Part print with two shaded views. Sizes in mm from the minimum x, y, z corner. A direction names the side the tool comes from. Round coordinates to 2 decimals unless told otherwise and drop trailing zeros. Loops run counter-clockwise (first coordinate to the right, second up) from the corner with the lowest first, then second, coordinate; pieces in that order, holes last. Notation, with made-up numbers: M 23,79 L 33,79 A27 cw 33,112 Z; hole C -23.75,30 d5. An arc over 180 degrees is marked long. Use a Markdown table: item, result. Add a question column.
Item 1: Saw through at D-D on x = 1.5. Write the cut outline in (y, z).
Item 2: Saw through at C-C on x = 0.5. Write the cut outline in (y, z).
Item 3: Tool access for the marked faces 1, 2 and 3: list every direction of +Z, -Z, +X, -X, +Y, -Y with a clear straight run to the whole face (end or side of a thin tool).
Item 4: Saw through at A-A on y = 4. Write the cut outline in (x, z).
Item 5: Pin check, flat tips, straight feed: P1, Ø1.5, axis at x = 3, z = 7, coming from the +Y side; P2, Ø1.5, axis at x = 3.5, z = 2, coming from the +Y side; P3, Ø3.5, axis at y = 4, z = 3.5, coming from the -X side. Stop position of each tip, or through.
Item 6: Wall check: L1, parallel to Z at x = 7.65, y = 4; L2, parallel to Z at x = 1.75, y = 4; L3, parallel to Y at x = 6.5, z = 6 (1 decimal). Give the ranges that are in metal, low to high. Write a range as from..to.
Item 7: Two-plate mould, pull along Y, no slides. Class the marked faces 4, 5 and 6: +Y half, -Y half, draft (parallel to the pull), parting line (faces both ways), or undercut.
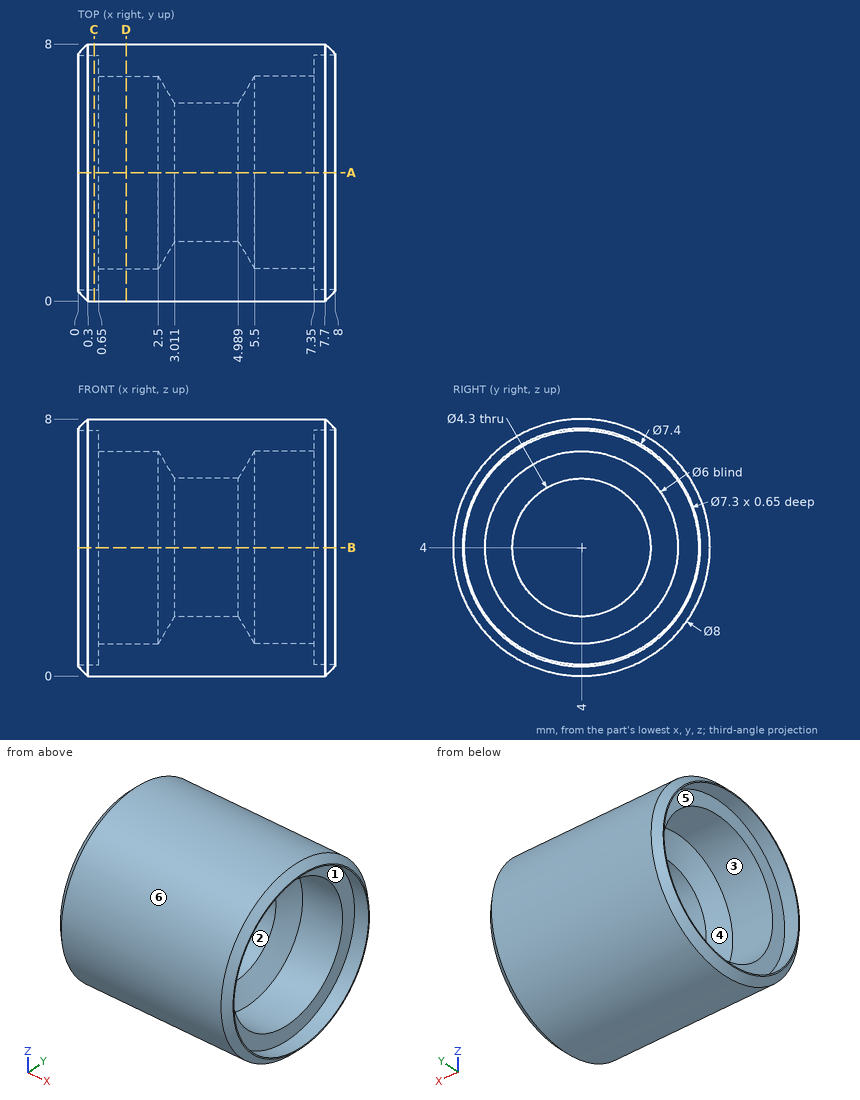
Entries:
| question | item | result |
|---|---|---|
| 1 | outline | C 4,4 d8; hole C 4,4 d6 |
| 2 | outline | C 4,4 d8; hole C 4,4 d7.3 |
| 3 | face 1 | +X |
| 3 | face 2 | +X, -X |
| 3 | face 3 | -X |
| 4 | outline | M 0,0.3 L 0.3,0 L 7.7,0 L 8,0.3 L 8,0.35 L 7.35,0.35 L 7.35,1 L 5.5,1 L 4.99,1.85 L 3.01,1.85 L 2.5,1 L 0.65,1 L 0.65,0.35 L 0,0.35 Z; M 0,7.65 L 0.65,7.65 L 0.65,7 L 2.5,7 L 3.01,6.15 L 4.99,6.15 L 5.5,7 L 7.35,7 L 7.35,7.65 L 8,7.65 L 8,7.7 L 7.7,8 L 0.3,8 L 0,7.7 Z |
| 5 | P1 | y = 7.31 |
| 5 | P2 | y = 7.8 |
| 5 | P3 | x = 2.95 |
| 6 | L1 | 0..0.35, 7.65..8 |
| 6 | L2 | 0..1, 7..8 |
| 6 | L3 | 0.5..1.8, 6.2..7.5 |
| 7 | face 4 | undercut |
| 7 | face 5 | undercut |
| 7 | face 6 | parting line |
